Work out the finished part from the listing and answer in its coordinate system (mm). Face numbers are marked on the shaded views. Round coordinates to 2 decimals unless told otherwise and drop trailing zeros. Loops run counter-clockwise (first coordinate to the right, second up) from the corner with the lowest first, then second, coordinate; pieces in that order, holes last. Notation, with made-up numbers: (40.5, 26.25) - (49.5, 26.25) arc R20 ccw to (49.5, 51.25) - close; hole circle Ø10 at (46.25, 12). An arc over 180 degrees is marked (long way). Answer as CSV lines item,"result". Start each with the question number.
```python
from build123d import *

# Parameters (mm, degrees)
SKETCH1_R           = 3.3782
BOSS_EXTRUDE1_DEPTH = 3.175


with BuildPart() as part:
    # Sketch1 → Boss-Extrude1 (new body)
    with BuildSketch(Plane.XY):
        with BuildLine():
            ThreePointArc((-104.047091932, -9.195763393), (-92.636784441, -3.320028798), (-97.435324623, 8.583474309))
            Line((-97.435324623, 8.583474309), (-128.331370442, 23.446143348))
            ThreePointArc((-128.331370442, 23.446143348), (-121.933316865, 7.574805873), (-137.147060186, -0.259506921))
            Line((-137.147060186, -0.259506921), (-104.047091932, -9.195763393))
        make_face()
        with Locations((-101.56444, 0)):
            Circle(SKETCH1_R, mode=Mode.SUBTRACT)
    extrude(amount=BOSS_EXTRUDE1_DEPTH)


solid = part.part
```
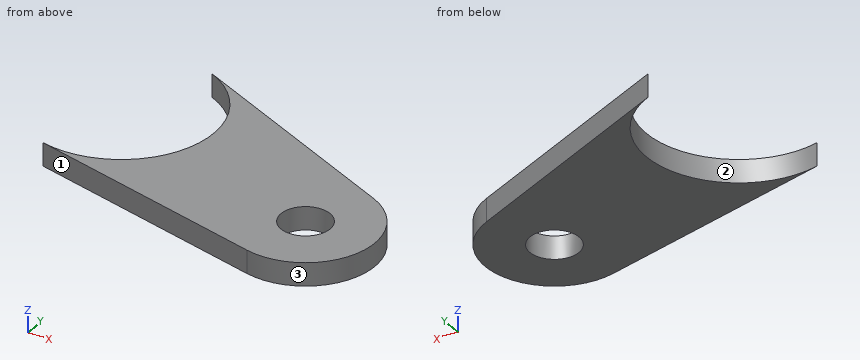
Item 1: Determine the mould class of the marked faces 1, 2 and 3 for opening direction Y: pulls with the +Y half, pulls with the -Y half, needs draft (parallel to the pull), parting line crosses it, or undercut.
Item 2: Section D-D, the plane y = 19 is taken. Give the vertices of the cut face in (x, z) (3 decimals), and give its area (3 significant figures).
Item 3: Find the intervals of material crossed by L1, parallel to Y at x = -101.5, z = 0.85; L2, parallel to Y at x = -122.5, z = 1.55; L3, parallel to X at y = 6.5, z = 0.2, in increasing order.
Item 4: Section B-B, the plane x = -100 is taken. Give the vertices of the cut face in (y, z) (3 decimals).
Item 5: Section C-C, the plane y = 2 is taken. Give the vertices of the cut face in (x, z) (3 decimals), and give its area (3 significant figures).
Answer:
1,face 1,"pulls with the -Y half"
1,face 2,"undercut"
1,face 3,"parting line crosses it"
2,outline,"(-123.239, 0) - (-119.089, 0) - (-119.089, 3.175) - (-123.239, 3.175) - close"
2,area,"13.2 mm²"
3,L1,"y = -9.52 to -3.38, 3.38 to 10.54"
3,L2,"y = -4.21 to 6.28, 17.73 to 20.64"
3,L3,"x = -122.39 to -94.6"
4,outline,"(-9.396, 0) - (-2.994, 0) - (-2.994, 3.175) - (-9.396, 3.175) - close; (2.994, 0) - (9.817, 0) - (9.817, 3.175) - (2.994, 3.175) - close"
5,outline,"(-126.01, 0) - (-104.287, 0) - (-104.287, 3.175) - (-126.01, 3.175) - close; (-98.842, 0) - (-92.252, 0) - (-92.252, 3.175) - (-98.842, 3.175) - close"
5,area,"89.9 mm²"
